CAD build for the part. Positions are in the model's coordinates, mm. A direction names the side the tool comes from. Coordinates: 2 decimals unless noted, no trailing zeros. Loops run counter-clockwise (first coordinate to the right, second up) from the corner with the lowest first, then second, coordinate; pieces in that order, holes last. Notation, with made-up numbers: (18.25, 53.25) -> (42.25, 53.25) arc R14 cw to (42.25, 63.25) -> close; hole circle Ø11 at (59, 87). An arc over 180 degrees is marked (long way). Answer as a JSON object with one key per item and string values. Group by question number.
from build123d import *

# Parameters (mm, degrees)
SKETCH1_W           = 7.6
SKETCH1_H           = 20.4
BOSS_EXTRUDE1_DEPTH = 10
SKETCH2_W           = 12
SKETCH2_H           = 24
BOSS_EXTRUDE2_DEPTH = 1.5
BOSS_EXTRUDE3_DEPTH = 7.7
FILLET1_R           = 1


with BuildPart() as part:
    # Sketch1 → Boss-Extrude1 (new body)
    with BuildSketch(Plane.XY):
        Rectangle(SKETCH1_W, SKETCH1_H)
    extrude(amount=BOSS_EXTRUDE1_DEPTH)

    # Sketch2 → Boss-Extrude2 (add)
    with BuildSketch(Plane.XY.offset(10)):
        Rectangle(SKETCH2_W, SKETCH2_H)
    extrude(amount=BOSS_EXTRUDE2_DEPTH)

    # Sketch3 → Boss-Extrude3 (add)
    with BuildSketch(Plane(origin=(3.8, 0, 0), x_dir=(0, 0, -1), z_dir=(1, 0, 0))):
        Polygon((-11.5, 7), (-14.5, 7), (-12.604811218, 0), (-14.5, -7), (-11.5, -7), align=None)
    extrude(amount=-BOSS_EXTRUDE3_DEPTH)

    # Fillet1
    fillet1_edges = [part.edges().sort_by_distance(p)[0] for p in [
        (-0.05, -7, 14.5),
        (-0.05, 7, 14.5),
    ]]
    fillet(fillet1_edges, radius=FILLET1_R)


solid = part.part
Item 1: Band-saw the part on A-A, the plane y = 8.5. List the corners of the cut face in (x, z).
Item 2: Band-saw the part on D-D, the plane y = -1.75. List the corners of the cut face in (x, z).
Item 3: Drill centre lines: L1, parallel to Z at x = 0.25, y = -7.75; L2, parallel to Z at x = 4.5, y = -2; L3, parallel to X at y = -4.5, z = 2.75. Where is each one in solid material? Low to high.
Item 4: Pull direction Y, two halves, no side cores. Call faces 5 (the flat face through (0, -10.2, 5)), 6 (the flat face through (0.004, 2.91, 13.393)), 7 (the flat face through (-4.1, 0.2, 11.5)): +Y half, -Y half, draft (parallel to the pull), parting line (faces both ways), or undercut.
Item 5: Band-saw the part on C-C, the plane z = 12.25. List the corners of the cut face in (x, y), and give its area (3 significant figures).
Item 6: 3-axis set-ups, long thin cutter, end or side, ignore diameter. For faces 1 (the flat face through (-3.8, 0, 5)), 2 (the flat face through (0, -2.83, 13.37)), 3 (the flat face through (0, -7, 12)), 4 (the flat face through (3.8, 0, 5)): which of +Z, -Z, +X, -X, +Y, -Y reach the whole face in a straight line?
Item 7: Flat gauge pins, fed straight in: P1, Ø0.8, axis at y = -2.5, z = 12.5, coming from the +X side; P2, Ø5, axis at x = -4, y = 0, coming from the +Z side; P3, Ø8, axis at y = -4.5, z = 4, coming from the -X side. Where does each tip first touch, or does it go through?
Item 8: Band-saw the part on B-B, the plane x = -0.5. List the corners of the cut face in (y, z), and give its area (3 significant figures).
Reply:
{
 "1": {"outline": "(-6, 10) -> (-3.8, 10) -> (-3.8, 0) -> (3.8, 0) -> (3.8, 10) -> (6, 10) -> (6, 11.5) -> (-6, 11.5) -> close"},
 "2": {"outline": "(-6, 10) -> (-3.8, 10) -> (-3.8, 0) -> (3.8, 0) -> (3.8, 10) -> (6, 10) -> (6, 11.5) -> (3.8, 11.5) -> (3.8, 13.08) -> (-3.9, 13.08) -> (-3.9, 11.5) -> (-6, 11.5) -> close"},
 "3": {"L1": "0 to 11.5", "L2": "10 to 11.5", "L3": "-3.8 to 3.8"},
 "4": {"face 5": "-Y half", "face 6": "undercut", "face 7": "draft"},
 "5": {"outline": "(-3.9, -7) -> (3.8, -7) -> (3.8, 7) -> (-3.9, 7) -> close", "area": "108 mm²"},
 "6": {"face 1": "-Z, -X, +Y, -Y", "face 2": "+Z, +X, -X", "face 3": "+Z, +X, -X, -Y", "face 4": "-Z, +X, +Y, -Y"},
 "7": {"P1": "x = 3.8", "P2": "z = 13.28", "P3": "x = -3.8"},
 "8": {"outline": "(-12, 10) -> (-10.2, 10) -> (-10.2, 0) -> (10.2, 0) -> (10.2, 10) -> (12, 10) -> (12, 11.5) -> (7, 11.5) -> (7, 13.19) arc R1 ccw to (5.74, 14.16) -> (0, 12.6) -> (-5.74, 14.16) arc R1 ccw to (-7, 13.19) -> (-7, 11.5) -> (-12, 11.5) -> close", "area": "268 mm²"}
}
